Can you work these out from the model? Positions are in its coordinate system, mm. Face numbers are marked on the shaded views. A direction names the side the tool comes from. Round coordinates to 2 decimals unless told otherwise and drop trailing zeros. Loops run counter-clockwise (first coordinate to the right, second up) from the corner with the lowest first, then second, coordinate; pieces in that order, holes last. Notation, with made-up numbers: M 9,12.5 L 36,12.5 A34 ccw 36,50.5 Z; hole C 80.5,17.25 d3. An arc over 180 degrees is marked long. Return JSON: item names as keys, results as strings.
```python
from build123d import *

# Parameters (mm, degrees)
SKETCH2_R           = 49.5
SKETCH2_W           = 5.44
SKETCH2_H           = 15
BOSS_EXTRUDE1_DEPTH = 7
BOSS_EXTRUDE2_START = 7
SKETCH2_3_W         = 115.8532
SKETCH2_3_H         = 25.8601
SKETCH2_3_W_2       = 11.343
SKETCH2_3_H_2       = 20.901
BOSS_EXTRUDE2_DEPTH = 25.4


with BuildPart() as part:
    # Sketch2 → Boss-Extrude1 (new body)
    with BuildSketch(Plane.XY):
        Polygon((-58.1817, 74.5), (-58.1817, 48.6399), (-56, 48.6399), (-56, -44), (-23, -77), (23, -77), (56, -44), (56, 48.6399), (57.6715, 48.6399), (57.6715, 74.5), align=None)
        Circle(SKETCH2_R, mode=Mode.SUBTRACT)
        with Locations((-16.5102, -63.2904)):
            Rectangle(SKETCH2_W, SKETCH2_H, mode=Mode.SUBTRACT)
        with Locations((-30.5102, 61.0904)):
            Rectangle(SKETCH2_W, SKETCH2_H, mode=Mode.SUBTRACT)
        with Locations((-49.5102, 61.0904)):
            Rectangle(SKETCH2_W, SKETCH2_H, mode=Mode.SUBTRACT)
        with Locations((-11.5102, 61.0904)):
            Rectangle(SKETCH2_W, SKETCH2_H, mode=Mode.SUBTRACT)
        with Locations((49, 61.0904)):
            Rectangle(SKETCH2_W, SKETCH2_H, mode=Mode.SUBTRACT)
        with Locations((30, 61.0904)):
            Rectangle(SKETCH2_W, SKETCH2_H, mode=Mode.SUBTRACT)
        with Locations((11, 61.0904)):
            Rectangle(SKETCH2_W, SKETCH2_H, mode=Mode.SUBTRACT)
        with Locations((-0.5102, -63.2904)):
            Rectangle(SKETCH2_W, SKETCH2_H, mode=Mode.SUBTRACT)
        with Locations((15.4898, -63.2904)):
            Rectangle(SKETCH2_W, SKETCH2_H, mode=Mode.SUBTRACT)
    extrude(amount=BOSS_EXTRUDE1_DEPTH)

    # Sketch2<3> → Boss-Extrude2 (add)
    # profile 1 of 2: a face of its own
    with BuildSketch(Plane.XY.offset(BOSS_EXTRUDE2_START)):
        with Locations((-0.2551, 61.56995)):
            Rectangle(SKETCH2_3_W, SKETCH2_3_H)
        with Locations((49, 61.0904)):
            Rectangle(SKETCH2_3_W_2, SKETCH2_3_H_2, mode=Mode.SUBTRACT)
        with Locations((-49.5102, 61.0904)):
            Rectangle(SKETCH2_3_W_2, SKETCH2_3_H_2, mode=Mode.SUBTRACT)
        with Locations((-30.5102, 61.0904)):
            Rectangle(SKETCH2_3_W_2, SKETCH2_3_H_2, mode=Mode.SUBTRACT)
        with Locations((-11.5102, 61.0904)):
            Rectangle(SKETCH2_3_W_2, SKETCH2_3_H_2, mode=Mode.SUBTRACT)
        with Locations((11, 61.0904)):
            Rectangle(SKETCH2_3_W_2, SKETCH2_3_H_2, mode=Mode.SUBTRACT)
        with Locations((30, 61.0904)):
            Rectangle(SKETCH2_3_W_2, SKETCH2_3_H_2, mode=Mode.SUBTRACT)
    # profile 2 of 2: a face of its own
    with BuildSketch(Plane.XY.offset(BOSS_EXTRUDE2_START)):
        Polygon((-25.1817, -49.8399), (-25.1817, -74.8183), (-23, -77), (23, -77), (24.1613, -75.8387), (24.1613, -49.8399), align=None)
        with Locations((-16.5102, -63.2904)):
            Rectangle(SKETCH2_3_W_2, SKETCH2_3_H_2, mode=Mode.SUBTRACT)
        with Locations((-0.5102, -63.2904)):
            Rectangle(SKETCH2_3_W_2, SKETCH2_3_H_2, mode=Mode.SUBTRACT)
        with Locations((15.4898, -63.2904)):
            Rectangle(SKETCH2_3_W_2, SKETCH2_3_H_2, mode=Mode.SUBTRACT)
    extrude(amount=BOSS_EXTRUDE2_DEPTH)


solid = part.part
```
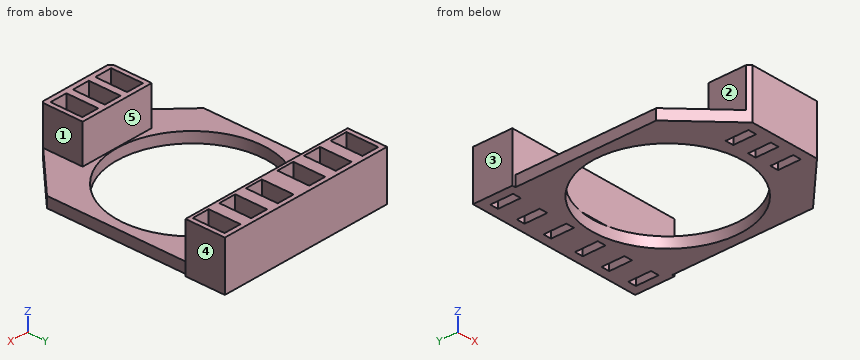
Q1. Suppose I cut it at A-A, the plane y = 0. Please give me the cut outline in (x, z), plus the area to 3 significant figures.
Results:
{"outline": "M -56,0 L -49.5,0 L -49.5,7 L -56,7 Z; M 49.5,0 L 56,0 L 56,7 L 49.5,7 Z", "area": "91.0 mm2"}
Q2. I'm going to push flat-ended pins straight in: pin 1 Ø10 at (x, y) = (-20.5, 40) entering from -Z; pin 2 Ø3.5 at (x, y) = (-14.5, -63) entering from +Z; pin 3 Ø5.5 at (y, z) = (23, 4) entering from +X; pin 4 Ø3.5 at (x, z) = (-47, 22) entering from -Y. Where does each tip first touch, or does it pass through?
Results:
{"pin 1": "stops at z = 0", "pin 2": "stops at z = 7", "pin 3": "stops at x = 56", "pin 4": "stops at y = 48.64"}
Q3. Suppose I cut it at B-B, the plane x = 0. Please give me the cut outline in (y, z), plus the area to 3 significant figures.
Results:
{"outline": "M -77,0 L -70.79,0 L -70.79,7 L -73.74,7 L -73.74,32.4 L -77,32.4 Z; M -55.79,0 L -49.5,0 L -49.5,7 L -49.84,7 L -49.84,32.4 L -52.84,32.4 L -52.84,7 L -55.79,7 Z; M 48.64,7 L 49.5,7 L 49.5,0 L 74.5,0 L 74.5,32.4 L 48.64,32.4 Z", "area": "1,080 mm2"}
Q4. If I drill on line 1 along Y through (x, z) = (0, 4); line 2 along Y through (x, z) = (11.5, 20); line 3 along Y through (x, z) = (-6.5, 17), over which ranges is the centre line in solid material (lowest first)?
Results:
{"line 1": "y = -77 to -70.79, -55.79 to -49.5, 49.5 to 74.5", "line 2": "y = -77 to -73.74, -52.84 to -49.84, 48.64 to 50.64, 71.54 to 74.5", "line 3": "y = -77 to -49.84, 48.64 to 50.64, 71.54 to 74.5"}
Q5. Suppose I cut it at C-C, the plane z = 17. State how many separate pieces and enclosed holes the cut face has, plus the area to 3 significant figures.
Results:
{"separate pieces": "2", "enclosed holes": "9", "area": "2,200 mm2"}
Q6. On a 3-axis mill with a long thin cutter (end or side, diameter ignored), from which of +Z, -Z, +X, -X, +Y, -Y can I reach the whole of each face in a straight line? I mean the marked faces 1, 2, 3, 4 and 5. Say none if no direction works.
Results:
{"face 1": "+Z, +X, -Y", "face 2": "+Z, -X, -Y", "face 3": "+Z, -Z, -X, +Y, -Y", "face 4": "+Z, -Z, +X, +Y, -Y", "face 5": "+Z, +X, -X"}
